Can you work these out from the model? Positions are in its coordinate system, mm. Face numbers are marked on the shaded views. A direction names the side the tool comes from. Coordinates: 2 decimals unless noted, no trailing zeros. Order: outer loops, then holes, each group sorted by start corner. A loop starts at its lowest first (then second) coordinate and runs counter-clockwise, first axis right, second up. Notation, with made-up numbers: (6.5, 63) -> (15.5, 63) arc R31 cw to (15.5, 90) -> close; hole circle Ø9 at (-14.75, 29). An arc over 180 degrees is marked (long way). Answer in a Markdown table with one row per item.
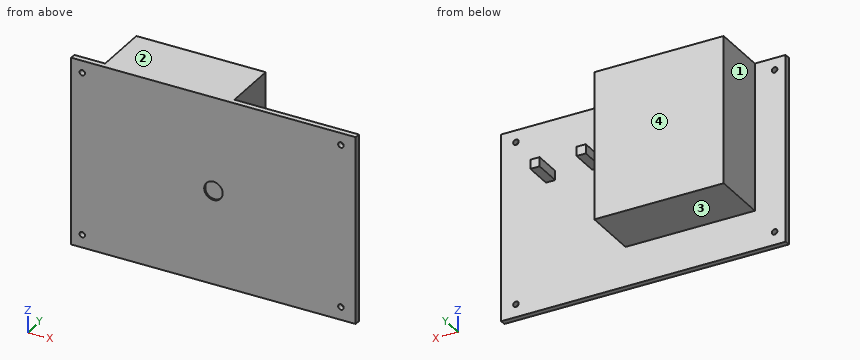
```python
from build123d import *

# Parameters (mm, degrees)
ESQUISSE1_W             = 154
ESQUISSE1_H             = 101.5
BOSS_EXTRU_1_DEPTH      = 3
ESQUISSE2_R             = 1.5
ENL_V_MAT_EXTRU_1_DEPTH = 3
ESQUISSE3_W             = 70
ESQUISSE3_H             = 80
BOSS_EXTRU_2_DEPTH      = 30
ESQUISSE4_W             = 5
ESQUISSE4_H             = 5
BOSS_EXTRU_3_DEPTH      = 15
ESQUISSE5_R             = 5
ENL_V_MAT_EXTRU_2_DEPTH = 1


with BuildPart() as part:
    # Esquisse1 → Boss.-Extru.1 (new body)
    with BuildSketch(Plane(origin=(0, 0, 0), x_dir=(1, 0, 0), z_dir=(0, 1, 0))):
        Rectangle(ESQUISSE1_W, ESQUISSE1_H)
    extrude(amount=BOSS_EXTRU_1_DEPTH)

    # Esquisse2 → Enlèv. mat.-Extru.1 (cut)
    with BuildSketch(Plane(origin=(0, 3, 0), x_dir=(1, 0, 0), z_dir=(0, 1, 0))):
        with Locations((-71, 43.75)):
            Circle(ESQUISSE2_R)
        with Locations((69, 43.75)):
            Circle(ESQUISSE2_R)
        with Locations((-71, -44.25)):
            Circle(ESQUISSE2_R)
        with Locations((69, -44.25)):
            Circle(ESQUISSE2_R)
    extrude(amount=-ENL_V_MAT_EXTRU_1_DEPTH, mode=Mode.SUBTRACT)

    # Esquisse3 → Boss.-Extru.2 (add)
    with BuildSketch(Plane(origin=(0, 3, 0), x_dir=(1, 0, 0), z_dir=(0, 1, 0))):
        with Locations((-25.3, -10.75)):
            Rectangle(ESQUISSE3_W, ESQUISSE3_H)
    extrude(amount=BOSS_EXTRU_2_DEPTH)

    # Esquisse4 → Boss.-Extru.3 (add)
    with BuildSketch(Plane(origin=(0, 3, 0), x_dir=(1, 0, 0), z_dir=(0, 1, 0))):
        with Locations((25.25, -20.25)):
            Rectangle(ESQUISSE4_W, ESQUISSE4_H)
        with Locations((50.25, -20.25)):
            Rectangle(ESQUISSE4_W, ESQUISSE4_H)
    extrude(amount=BOSS_EXTRU_3_DEPTH)

    # Esquisse5 → Enlèv. mat.-Extru.2 (cut)
    with BuildSketch(Plane.XZ):
        Circle(ESQUISSE5_R)
    extrude(amount=-ENL_V_MAT_EXTRU_2_DEPTH, mode=Mode.SUBTRACT)


solid = part.part
```
(1) Will these pins go through, and if not, where does the flat tip stop? pin 1 Ø4 at (x, y) = (51, 13) entering from +Z; pin 2 Ø1.5 at (y, z) = (23, -13) entering from +X; pin 3 Ø4 at (y, z) = (18.5, -8) entering from -X.
Response values:
| item | result |
|---|---|
| pin 1 | z = 22.75 |
| pin 2 | x = 9.7 |
| pin 3 | x = -60.3 |
(2) Suppose I cut it at D-D (z = 0). Please give me the cut outline in (x, y), and give its area (3 significant figures).
Response values:
| item | result |
|---|---|
| outline | (-77, 0) -> (-5, 0) -> (-5, 1) -> (5, 1) -> (5, 0) -> (77, 0) -> (77, 3) -> (9.7, 3) -> (9.7, 33) -> (-60.3, 33) -> (-60.3, 3) -> (-77, 3) -> close |
| area | 2,550 mm2 |
(3) On a 3-axis mill with a long thin cutter (end or side, diameter ignored), from which of +Z, -Z, +X, -X, +Y, -Y can I reach the whole of each face in a straight line? I mean the marked faces 3 and 4. Say none if no direction works.
Response values:
| item | result |
|---|---|
| face 3 | -Z, +X, -X, +Y |
| face 4 | +Z, -Z, +X, -X, +Y |
(4) I need wall thicknesses on line 1 (Z direction, x = 69, y = 1.55); line 2 (X direction, y = 0.7, z = -43.75); line 3 (X direction, y = 2, z = -43). Which ranges of each line are inside material? Lowest first, please. Write a range as [from, to].
Response values:
| item | result |
|---|---|
| line 1 | [-50.75, -45.25], [-42.25, 42.75], [45.75, 50.75] |
| line 2 | [-77, -72.5], [-69.5, 67.5], [70.5, 77] |
| line 3 | [-77, -72.3], [-69.7, 67.7], [70.3, 77] |
(5) Suppose I cut it at C-C (z = 44.25). Please give me the cut outline in (x, y), and give its area (3 significant figures).
Response values:
| item | result |
|---|---|
| outline | (-77, 0) -> (-72.5, 0) -> (-72.5, 3) -> (-77, 3) -> close; (-69.5, 0) -> (67.5, 0) -> (67.5, 3) -> (9.7, 3) -> (9.7, 33) -> (-60.3, 33) -> (-60.3, 3) -> (-69.5, 3) -> close; (70.5, 0) -> (77, 0) -> (77, 3) -> (70.5, 3) -> close |
| area | 2,540 mm2 |
(6) Suppose I cut it at A-A (x = 69). Please give me the cut outline in (y, z), and give its area (4 significant figures).
Response values:
| item | result |
|---|---|
| outline | (0, -50.75) -> (3, -50.75) -> (3, -45.25) -> (0, -45.25) -> close; (0, -42.25) -> (3, -42.25) -> (3, 42.75) -> (0, 42.75) -> close; (0, 45.75) -> (3, 45.75) -> (3, 50.75) -> (0, 50.75) -> close |
| area | 286.5 mm2 |
(7) We'd pull the mould along X, two halves only. Please class the marked faces 1 and 2: +X half, -X half, draft (parallel to the pull), parting line (faces both ways), or undercut.
Response values:
| item | result |
|---|---|
| face 1 | -X half |
| face 2 | draft |
(8) Suppose I cut it at B-B (y = 10). Please give me the cut outline in (x, z), and give its area (3 significant figures).
Response values:
| item | result |
|---|---|
| outline | (-60.3, -29.25) -> (9.7, -29.25) -> (9.7, 50.75) -> (-60.3, 50.75) -> close; (22.75, 17.75) -> (27.75, 17.75) -> (27.75, 22.75) -> (22.75, 22.75) -> close; (47.75, 17.75) -> (52.75, 17.75) -> (52.75, 22.75) -> (47.75, 22.75) -> close |
| area | 5,650 mm2 |
